Part model, mm, in its own coordinate system. A direction names the side the tool comes from. Coordinates: 2 decimals unless noted, no trailing zeros. Loops run counter-clockwise (first coordinate to the right, second up) from the corner with the lowest first, then second, coordinate; pieces in that order, holes last. Notation, with made-up numbers: M -16,-10.5 L 1,-10.5 A17 cw 1,22.5 Z; hole C -13.75,-23 d11. An arc over 180 degrees is marked long. Answer as a JSON object with one key per item and string values. Group by question number.
1. Drop flat-ended pins along their axis: pin 1 Ø1.5 at (x, y) = (-22.5, 6) entering from +Z; pin 2 Ø1.3 at (x, y) = (-32.5, 3.5) entering from +Z; pin 3 Ø9.5 at (x, z) = (0, -33) entering from +Y. Give the stop position or say it passes through.
2. Mould opens along Z. For faces 4 (the face through (-35, 4, -26)), 5 (the face through (-41.764, 3.944, -28.883)), 6 (the face through (-21, 0, -28)) say: released by +Z, released by -Z, zero draft, split by the parting line, or undercut.
3. Saw through at B-B on x = -26.5. Write the cut outline in (y, z).
4. Saw through at A-A on y = 5.25. Count the separate pieces of the cut face and the enclosed holes in it, then the cut area to 3 significant figures.
5. Drill centre lines: L1, parallel to X at y = 1.5, z = -31.5; L2, parallel to Z at x = -15, y = 0.75; L3, parallel to Z at x = -25, y = 3.25. Where is each one in solid material? Low to high.
6. Saw through at C-C on z = -33. Write the cut outline in (x, y), then the cut area to 3 significant figures.
7. 3-axis set-ups, long thin cutter, end or side, ignore diameter. For faces 1 (the face through (-27, 4, -26.693)), 2 (the face through (-17, 4, -23)), 3 (the face through (-19, 7, -33)): which of +Z, -Z, +X, -X, +Y, -Y reach the whole face in a straight line?
Autodesk Inventor part; units mm, degrees
ref_plane "YZ Plane" through (0, 0, 0) normal (1, 0, 0) x (0, 1, 0)
ref_plane "XZ Plane" through (0, 0, 0) normal (0, 1, 0) x (-1, 0, 0)
ref_plane "XY Plane" through (0, 0, 0) normal (0, 0, 1) x (1, 0, 0)
sketch "Boceto1" plane through (0, 0, 0) normal (0, 1, 0) x (-1, 0, 0)
  line L0 (50, -16.5) -> (49.0807, -16.5)
  circle A0 centre (0, -33) radius 1.5
  circle A1 centre (0, -33) radius 3
  arc A2 (0, -26) -> (5.7446, -37) centre (0, -33) ccw
  line L1 (5.7446, -37) -> (35, -37)
  line L2 (35, -37) -> (50, -19)
  line L3 (0, -23) -> (20, -23)
  line L4 (20, -23) -> (20, -17)
  line L5 (20, -17) -> (50, -17)
  line L6 (50, -17) -> (50, -19)
  line L7 (0, -31.5) -> (0, -30)
  line L8 (0, -26) -> (0, -23)
  point P0 (0, -37)
extrude "Extrusión1" add sketch "Boceto1" along normal blind 8 contours A1 | L8 L3 L4 L5 L6 L2 L1 A2
sketch "Boceto2" plane through (0, 8, 0) normal (0, 1, 0) x (1, 0, 0)
  circle A0 centre (0, 0) radius 3
  dimension "d12" = 6
extrude "Extrusión2" cut sketch "Boceto2" against normal blind 4
sketch "Boceto6" plane through (0, 0, 0) normal (0, -1, 0) x (1, 0, 0)
  line L0 (-50, -17) -> (-20, -17)
  line L1 (-50, -16) -> (-50, -14)
  line L2 (-50, -17) -> (-50, -16)
  line L3 (-50, -16.5) -> (-16.403, -16.5)
  line L4 (-20, -23) -> (-25, -23)
  line L5 (-5.7446, -37) -> (-35, -37)
  line L6 (-25, -23) -> (-25, -28)
  line L7 (-25, -37) -> (-25, -32)
  line L8 (-25, -32) -> (-5.7446, -32)
  line L9 (-5.7446, -32) -> (-5.7446, -27.061)
  line L10 (-25, -28) -> (-5.7446, -28)
  line L11 (-35, -37) -> (-30, -37)
  line L12 (-30, -37) -> (-30, -32)
  line L13 (-30, -32) -> (-25, -32)
  line L14 (-50, -19) -> (-50, -17)
  line L15 (-50, -19) -> (-45, -19)
  line L16 (-30, -37) -> (-45, -19)
  line L17 (-45, -19) -> (-40, -19)
  line L18 (-30, -32) -> (-40.8333, -19)
  line L19 (-40.8333, -19) -> (-25, -19)
  line L20 (-25, -19) -> (-25, -28)
  line L21 (-30, -32) -> (-34.1667, -32)
  line L22 (-40.8333, -19) -> (-35.8333, -19)
  line L23 (-35.8333, -19) -> (-25, -32)
  line L24 (-35.8333, -19) -> (-30.8333, -19)
  line L25 (-25, -32) -> (-20, -32)
  line L26 (-20, -32) -> (-30.8333, -19)
  line L27 (-30, 4) -> (-45, -14)
  line L28 (-45, -14) -> (-40, -14)
  line L29 (-30, -1) -> (-40.8333, -14)
  line L30 (-30, -1) -> (-34.1667, -1)
  line L31 (-35.8333, -14) -> (-25, -1)
  line L32 (-35.8333, -14) -> (-30.8333, -14)
  line L33 (-25, -1) -> (-20, -1)
  line L34 (-20, -1) -> (-30.8333, -14)
  point P0 (0, 0)
  dimension "d28" = 5
  dimension "d29" = 5
  dimension "d30" = 5
  dimension "d31" = 5
  dimension "d32" = 5
  dimension "d33" = 5
  dimension "d34" = 5
  dimension "d35" = 5
  dimension "d36" = 5
extrude "Extrusión6" cut sketch "Boceto6" against normal blind 10 contours L23 L19 L26 L6 L10 L8 | L21 L16 L17 L18 | L10 L6 L26 | L30 L29 L28 L27 | L31 L33 L34 L32
chamfer "Chaflán1" distance 2 angle 45 2 edges at (-50, 4, -19) (0, 4, -23)
sketch "Boceto9" plane through (0, 0, 0) normal (0, -1, 0) x (1, 0, 0)
  circle A0 centre (0, -33) radius 1.5
  circle A1 centre (0, -33) radius 3
  point P0 (0, 0)
  dimension "d47" = 6
extrude "Extrusión9" cut sketch "Boceto9" against normal blind 4
sketch "Boceto10" plane through (0, 8, 0) normal (0, 1, 0) x (1, 0, 0)
  circle A0 centre (0, 33) radius 1.5
  circle A1 centre (0, 33) radius 6
  line L0 (0, 33) -> (-19, 33)
  line L1 (0, 33) -> (0, 37.5)
  line L2 (0, 37.5) -> (-19, 37.5)
  line L3 (-19, 37.5) -> (-19, 28.5)
  line L4 (-19, 28.5) -> (0, 28.5)
  line L5 (-19, 33) -> (-16, 33)
  circle A2 centre (-16, 33) radius 3
  circle A3 centre (-16, 33) radius 3
  line L6 (-16, 36) -> (-3.9686, 37.5)
  line L7 (-16, 33) -> (-16, 30)
  line L8 (-16, 30) -> (-3.9686, 28.5)
  point P0 (0, 0)
  dimension "d50" = 12
  dimension "d51" = 19
  dimension "d52" = 4.5
  dimension "d53" = 9
  dimension "d54" = 3
extrude "Extrusión10" cut sketch "Boceto10" against normal blind 2 contours A0 L1 L2 A1 L0 | A0 L0 A1 L2 L1 | L0 A2 L6 A1 | A1 L8 A2 L0 | A2 L7 L0 | L0 A2 | A2 L0 L7
sketch "Boceto14" plane through (0, 0, 0) normal (0, -1, 0) x (1, 0, 0)
  line L0 (-40.8333, -14) -> (-30, -1)
  line L1 (-35.8333, -14) -> (-30.8333, -14)
  line L2 (-40.8333, -14) -> (-35.8333, -14)
  line L3 (-35.8333, -14) -> (-38.3333, -14)
  line L4 (-25, -1) -> (-35.8333, -14)
  line L5 (-35.8333, -14) -> (-29.4226, -6.3071)
  line L6 (-34.4226, -6.3071) -> (-29.4226, -6.3071)
  line L7 (-29.4226, -6.3071) -> (-20, -6.3071)
  line L8 (0, -10) -> (9, -10)
  line L9 (-20, -6.3071) -> (-20, -10)
  line L10 (-40.8333, -14) -> (-40.8333, -16)
  line L11 (-20, -16) -> (-50, -16)
  line L12 (-20, -10) -> (-20, -16)
  line L13 (-40.8333, -16) -> (-20, -16)
  line L14 (-20, -16) -> (-20, -10)
  line L15 (-35.8333, -14) -> (-30.8333, -14)
  line L16 (-30.8333, -14) -> (-20, -1)
  line L17 (-24.4226, -6.3071) -> (-30.8333, -14)
  line L18 (-35.8333, -14) -> (-40.8333, -16)
  line L19 (-50, -16) -> (-50, -17)
  line L20 (-50, -16.5) -> (-40.8333, -16.5)
  line L21 (-40.8333, -19) -> (-30, -32)
  line L22 (-35.8333, -19) -> (-30.8333, -19)
  line L23 (-40.8333, -19) -> (-35.8333, -19)
  line L24 (-35.8333, -19) -> (-38.3333, -19)
  line L25 (-25, -32) -> (-35.8333, -19)
  line L26 (-35.8333, -19) -> (-29.4226, -26.6929)
  line L27 (-34.4226, -26.6929) -> (-29.4226, -26.6929)
  line L28 (-29.4226, -26.6929) -> (-20, -26.6929)
  line L29 (-20, -26.6929) -> (-20, -23)
  line L30 (-40.8333, -19) -> (-40.8333, -17)
  line L31 (-20, -23) -> (-20, -17)
  line L32 (-40.8333, -17) -> (-20, -17)
  line L33 (-20, -17) -> (-20, -23)
  line L34 (-35.8333, -19) -> (-30.8333, -19)
  line L35 (-30.8333, -19) -> (-20, -32)
  line L36 (-24.4226, -26.6929) -> (-30.8333, -19)
  line L37 (-35.8333, -19) -> (-40.8333, -17)
  point P0 (0, 0)
  point P1 (7, -10)
extrude "Extrusión13" cut sketch "Boceto14" against normal blind 8 contours L18 L1 L16 L7 L9 L12 L11 | L32 L31 L29 L28 L35 L22 L37
sketch "Boceto15" plane through (0, 0, 0) normal (0, -1, 0) x (1, 0, 0)
  line L0 (-20, -6.3071) -> (-24.4226, -6.3071)
  line L1 (-20, -6.3071) -> (-29.4226, -6.3071)
  line L2 (-35.8333, -14) -> (-25, -1)
  line L3 (-20, -10) -> (-20, -6.3071)
  line L4 (-20, -10) -> (-32.5381, -10)
  line L5 (-32.5381, -10) -> (-29.4226, -6.3071)
  line L6 (-50, -17) -> (-40.8333, -17)
  line L7 (-40.8333, -16) -> (-50, -16)
  line L8 (-50, -17) -> (-50, -16)
  line L9 (-50, -16.5) -> (-36.6527, -16.5)
  line L10 (-20, -26.6929) -> (-24.4226, -26.6929)
  line L11 (-20, -26.6929) -> (-29.4226, -26.6929)
  line L12 (-20, -23) -> (-20, -26.6929)
  line L13 (-20, -23) -> (-32.5381, -23)
  line L14 (-32.5381, -23) -> (-29.4226, -26.6929)
  point P0 (0, 0)
  point P1 (-32.5, -10)
extrude "Extrusión14" add sketch "Boceto15" against normal blind 8 contours L3 L4 L2 L1 L0 | L10 L11 L14 L13 L12
sketch "Boceto17" plane through (0, 8, 0) normal (0, 1, 0) x (1, 0, 0)
  line L0 (-20, 10) -> (-32.5, 10)
  line L1 (-29.4226, 6.3071) -> (-20, 6.3071)
  line L2 (-32.5, 10) -> (-29.4226, 6.3071)
  line L3 (-29.4226, 6.3071) -> (-20, 6.3071)
  line L4 (-20, 6.3071) -> (-20, 10)
  line L5 (-20, 6.3071) -> (-20, 10)
  line L6 (-20, 10) -> (-32.5, 10)
  point P0 (0, 0)
extrude "Extrusión16" cut sketch "Boceto17" against normal blind 10
properties part number "signle v2"
Outcome:
{
 "1": {"pin 1": "stops at z = -23", "pin 2": "stops at z = -22.22", "pin 3": "stops at y = 6"},
 "2": {"face 4": "undercut", "face 5": "released by -Z", "face 6": "zero draft"},
 "3": {"outline": "M 0,-37 L 8,-37 L 8,-30.2 L 0,-30.2 Z; M 0,-26.69 L 8,-26.69 L 8,-23 L 0,-23 Z"},
 "4": {"separate pieces": "1", "enclosed holes": "3", "area": "650 mm²"},
 "5": {"L1": "x = -39.58 to -34.58, -30.42 to -25.42, -20.42 to -2.6, 2.6 to 6.84", "L2": "z = -37 to -23", "L3": "z = -37 to -32, -26.69 to -23"},
 "6": {"outline": "M -38.33,0 L -3,0 L -3,4 L -1.5,4 L -1.5,6 L -19,6 L -19,8 L -38.33,8 Z; M 1.5,4 L 3,4 L 3,0 L 7,0 L 7,8 L 6,8 L 6,6 L 1.5,6 Z", "area": "283 mm²"},
 "7": {"face 1": "+Y, -Y", "face 2": "+Z, +X, +Y, -Y", "face 3": "+Y"}
}
